Here's how the part is built. I have some questions about the finished solid (model axes, mm). Face numbers are marked on the shaded views. A direction names the side the tool comes from. Round coordinates to 2 decimals unless told otherwise and drop trailing zeros. Loops run counter-clockwise (first coordinate to the right, second up) from the corner with the lowest first, then second, coordinate; pieces in that order, holes last. Notation, with made-up numbers: M 48.25,52.25 L 75.25,52.25 A24 ccw 75.25,71.25 Z; hole C 47,3 d6. An arc over 180 degrees is marked long. Use a Markdown table: item, result.
Autodesk Fusion 360 part; units mm, degrees
sketch "Sketch1" plane through (0, 0, 0) normal (0, 0, 1) x (1, 0, 0)
sketch "Sketch2" plane through (0, 0, 0) normal (0, 0, 1) x (1, 0, 0)
  line L0 (106.508, 35.5843) -> (319.36, 35.5843)
  line L1 (106.508, 35.5843) -> (106.508, 50.8243)
  line L2 (106.508, 50.8243) -> (65.868, 50.8243)
  line L3 (65.868, 50.8243) -> (65.868, 177.8243)
  line L4 (65.868, 177.8243) -> (106.508, 177.8243)
  line L5 (106.508, 177.8243) -> (106.508, 251.4843)
  line L6 (106.508, 251.4843) -> (319.36, 251.4843)
  line L7 (319.36, 251.4843) -> (319.36, 236.2443)
  line L8 (319.36, 236.2443) -> (360, 236.2443)
  line L9 (360, 236.2443) -> (360, 109.2443)
  line L10 (360, 109.2443) -> (319.36, 109.2443)
  line L11 (319.36, 109.2443) -> (319.36, 35.5843)
  dimension "d2" = 212.852
  dimension "d3" = 15.24
  dimension "d4" = 40.64
  dimension "d5" = 127
  dimension "d6" = 40.64
  dimension "d7" = 73.66
  dimension "d8" = 212.852
  dimension "d9" = 15.24
  dimension "d10" = 40.64
  dimension "d11" = 73.66
extrude "Extrude1" add sketch "Sketch2" along normal blind 254
sketch "Sketch3" plane through (0, 0, 254) normal (0, 0, 1) x (-1, 0, 0)
  line L0 (-106.508, -35.5843) -> (-319.36, -35.5843)
  line L1 (-319.36, -35.5843) -> (-319.36, -109.2443)
  line L2 (-319.36, -109.2443) -> (-360, -109.2443)
  line L3 (-360, -109.2443) -> (-360, -236.2443)
  line L4 (-360, -236.2443) -> (-319.36, -236.2443)
  line L5 (-319.36, -236.2443) -> (-319.36, -251.4843)
  line L6 (-319.36, -251.4843) -> (-106.508, -251.4843)
  line L7 (-106.508, -251.4843) -> (-106.508, -177.8243)
  line L8 (-106.508, -177.8243) -> (-65.868, -177.8243)
  line L9 (-65.868, -177.8243) -> (-65.868, -50.8243)
  line L10 (-65.868, -50.8243) -> (-106.508, -50.8243)
  line L11 (-106.508, -50.8243) -> (-106.508, -35.5843)
  line L12 (-65.868, -177.8243) -> (-66.868, -177.8243)
  line L13 (-66.868, -177.8243) -> (-66.868, -50.8243)
  line L14 (-66.868, -50.8243) -> (-65.868, -50.8243)
  line L15 (-65.868, -50.8243) -> (-65.868, -177.8243)
  line L16 (-65.868, -177.8243) -> (-107.508, -177.8243)
  line L17 (-107.508, -177.8243) -> (-107.508, -176.8243)
  line L18 (-107.508, -176.8243) -> (-65.868, -176.8243)
  line L19 (-65.868, -176.8243) -> (-65.868, -177.8243)
  line L20 (-65.868, -50.8243) -> (-107.508, -50.8243)
  line L21 (-107.508, -50.8243) -> (-107.508, -51.8243)
  line L22 (-107.508, -51.8243) -> (-65.868, -51.8243)
  line L23 (-65.868, -51.8243) -> (-65.868, -50.8243)
  line L24 (-107.508, -51.8243) -> (-106.508, -51.8243)
  line L25 (-106.508, -51.8243) -> (-106.508, -35.5843)
  line L26 (-106.508, -35.5843) -> (-107.508, -35.5843)
  line L27 (-107.508, -35.5843) -> (-107.508, -51.8243)
  line L28 (-106.508, -35.5843) -> (-319.36, -35.5843)
  line L29 (-319.36, -35.5843) -> (-319.36, -36.5843)
  line L30 (-319.36, -36.5843) -> (-106.508, -36.5843)
  line L31 (-106.508, -36.5843) -> (-106.508, -35.5843)
  line L32 (-319.36, -35.5843) -> (-318.36, -35.5843)
  line L33 (-318.36, -35.5843) -> (-318.36, -110.2443)
  line L34 (-318.36, -110.2443) -> (-319.36, -110.2443)
  line L35 (-319.36, -110.2443) -> (-319.36, -35.5843)
  line L36 (-318.36, -110.2443) -> (-360, -110.2443)
  line L37 (-360, -110.2443) -> (-360, -109.2443)
  line L38 (-360, -109.2443) -> (-318.36, -109.2443)
  line L39 (-318.36, -109.2443) -> (-318.36, -110.2443)
  line L40 (-360, -236.2443) -> (-359, -236.2443)
  line L41 (-359, -236.2443) -> (-359, -109.2443)
  line L42 (-359, -109.2443) -> (-360, -109.2443)
  line L43 (-360, -109.2443) -> (-360, -236.2443)
  line L44 (-360, -236.2443) -> (-318.36, -236.2443)
  line L45 (-318.36, -236.2443) -> (-318.36, -235.2443)
  line L46 (-318.36, -235.2443) -> (-360, -235.2443)
  line L47 (-360, -235.2443) -> (-360, -236.2443)
  line L48 (-319.36, -251.4843) -> (-318.36, -251.4843)
  line L49 (-318.36, -251.4843) -> (-318.36, -235.2443)
  line L50 (-318.36, -235.2443) -> (-319.36, -235.2443)
  line L51 (-319.36, -235.2443) -> (-319.36, -251.4843)
  line L52 (-319.36, -251.4843) -> (-106.508, -251.4843)
  line L53 (-106.508, -251.4843) -> (-106.508, -250.4843)
  line L54 (-106.508, -250.4843) -> (-319.36, -250.4843)
  line L55 (-319.36, -250.4843) -> (-319.36, -251.4843)
  line L56 (-107.508, -176.8243) -> (-106.508, -176.8243)
  line L57 (-106.508, -176.8243) -> (-106.508, -251.4843)
  line L58 (-106.508, -251.4843) -> (-107.508, -251.4843)
  line L59 (-107.508, -251.4843) -> (-107.508, -176.8243)
  dimension "d14" = 1
  dimension "d15" = 1
  dimension "d16" = 1
  dimension "d17" = 1
  dimension "d18" = 1
  dimension "d19" = 1
  dimension "d20" = 1
  dimension "d21" = 1
  dimension "d22" = 1
  dimension "d23" = 1
  dimension "d24" = 1
  dimension "d25" = 1
extrude "Extrude2" add sketch "Sketch3" along normal blind 5 contours L0 L11 L25 L26 L27 L28 L30 L31 | L0 L27 L28 L30 L33 | L11 L20 L25 L27 L30 | L0 L1 L28 L29 L30 L32 L33 L35 | L20 L21 L22 L24 L25 L27 | L10 L13 L20 L22 L25 | L1 L30 L33 L35 L38 | L9 L10 L13 L14 L15 L20 L22 L23 | L33 L34 L35 L36 L38 L39 | L9 L13 L15 L18 L22 | L2 L35 L36 L38 L41 | L8 L9 L12 L13 L15 L16 L18 L19 | L8 L13 L16 L18 L57 | L2 L3 L36 L37 L38 L41 L42 L43 | L16 L17 L18 L56 L57 L59 | L3 L36 L41 L43 L46 | L7 L16 L54 L57 L59 | L4 L41 L44 L46 L51 | L3 L4 L40 L41 L43 L44 L46 L47 | L6 L7 L52 L53 L54 L57 L58 L59 | L44 L45 L46 L49 L50 L51 | L6 L49 L52 L54 L59 | L5 L44 L49 L51 L54 | L5 L6 L48 L49 L51 L52 L54 L55
sketch "Sketch4" plane through (0, 0, 254) normal (0, 0, 1) x (-1, 0, 0)
  line L0 (-107.508, -176.8243) -> (-66.868, -176.8243)
  line L1 (-66.868, -176.8243) -> (-66.868, -51.8243)
  line L2 (-66.868, -51.8243) -> (-107.508, -51.8243)
  line L3 (-107.508, -51.8243) -> (-107.508, -36.5843)
  line L4 (-107.508, -36.5843) -> (-318.36, -36.5843)
  line L5 (-318.36, -36.5843) -> (-318.36, -110.2443)
  line L6 (-318.36, -110.2443) -> (-359, -110.2443)
  line L7 (-359, -110.2443) -> (-359, -235.2443)
  line L8 (-359, -235.2443) -> (-318.36, -235.2443)
  line L9 (-318.36, -235.2443) -> (-318.36, -250.4843)
  line L10 (-318.36, -250.4843) -> (-107.508, -250.4843)
  line L11 (-107.508, -250.4843) -> (-107.508, -176.8243)
  line L12 (-192.7092, -113.2958) -> (-177.8821, -135.8603)
  line L13 (-177.8821, -135.8603) -> (-181.5924, -155.5132)
  line L14 (-181.5924, -155.5132) -> (-189.7272, -162.9176)
  line L15 (-189.7272, -162.9176) -> (-197.3239, -162.6933)
  line L16 (-197.3239, -162.6933) -> (-208.6768, -121.2191)
  line L17 (-208.6768, -121.2191) -> (-209.0766, -103.7236)
  line L18 (-209.0766, -103.7236) -> (-206.2382, -88.6892)
  dimension "d40" = 27
  dimension "d42" = 11
  dimension "d44" = 43
  dimension "d46" = 17.5
  dimension "d47" = 7.6
  dimension "d48" = 107
  dimension "d49" = 166
  dimension "d50" = 20
  dimension "d51" = 136
  dimension "d52" = 143
  dimension "d54" = 15.3
  dimension "d55" = 168
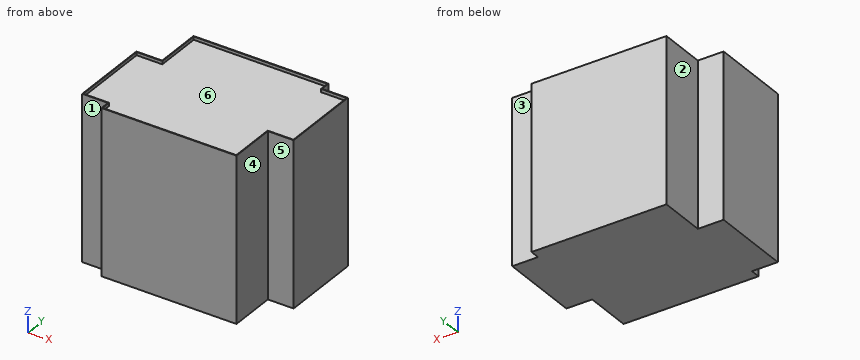
Q1. Imagine slicing it at A-A, the plane x = 236. Please give me the cut outline in (y, z), then the cut area to 3 significant figures.
Return value:
| item | result |
|---|---|
| outline | M 35.58,0 L 251.48,0 L 251.48,259 L 250.48,259 L 250.48,254 L 36.58,254 L 36.58,259 L 35.58,259 Z |
| area | 54,800 mm^2 |
Q2. I need wall thicknesses on line 1 (X direction, y = 233, z = 16); line 2 (Z direction, x = 199, y = 207); line 3 (Y direction, x = 320, z = 155.5). Which ranges of each line are inside material? Lowest first, please. Write a range as from..to.
Return value:
| item | result |
|---|---|
| line 1 | x = 106.51..360 |
| line 2 | z = 0..254 |
| line 3 | y = 109.24..236.24 |
Q3. Will these pins go through, and if not, where does the flat tip stop? P1, Ø4, axis at y = 43, z = 255.5, coming from the +X side; P2, Ø2.5, axis at x = 79, z = 256, coming from the +Y side; P3, Ø10, axis at y = 210, z = 101.5, coming from the -X side.
Return value:
| item | result |
|---|---|
| P1 | stops at x = 319.36 |
| P2 | stops at y = 177.82 |
| P3 | stops at x = 106.51 |
Q4. We'd pull the mould along X, two halves only. Please class the marked faces 4, 5 and 6: pulls with the +X half, pulls with the -X half, needs draft (parallel to the pull), parting line crosses it, or undercut.
Return value:
| item | result |
|---|---|
| face 4 | pulls with the +X half |
| face 5 | needs draft |
| face 6 | undercut |
Q5. Imagine slicing it at C-C, the plane z = 18. Please give me the cut outline in (x, y).
Return value:
| item | result |
|---|---|
| outline | M 65.87,50.82 L 106.51,50.82 L 106.51,35.58 L 319.36,35.58 L 319.36,109.24 L 360,109.24 L 360,236.24 L 319.36,236.24 L 319.36,251.48 L 106.51,251.48 L 106.51,177.82 L 65.87,177.82 Z |
Q6. Imagine slicing it at B-B, the plane y = 231. Please give me the cut outline in (x, z).
Return value:
| item | result |
|---|---|
| outline | M 106.51,0 L 360,0 L 360,259 L 359,259 L 359,254 L 107.51,254 L 107.51,259 L 106.51,259 Z |
Q7. For the marked faces 1, 2 and 3, which set-ups out of +Z, -Z, +X, -X, +Y, -Y let a thin tool reach every point of the face, with its end or its side?
Return value:
| item | result |
|---|---|
| face 1 | +Z, -Z, -X, -Y |
| face 2 | +Z, -Z, -X, +Y |
| face 3 | +Z, -Z, +X, +Y |
